Geometry: final body of the model. Coordinates: model frame, mm. A direction names the side the tool comes from. Give positions to 0.01 mm unless a question says otherwise; leave off trailing zeros. Write each loop counter-clockwise with the first axis right and the second up, starting at its lowest first coordinate (ties: lowest second). Pieces come first, ordered by that corner, then holes. Notation, with made-up numbers: (47, 41.5) -> (85, 41.5) arc R26 ccw to (85, 71.5) -> close; hole circle Ø8 at (-17.5, 33). An arc over 180 degrees is marked (long way). Answer in a Markdown table with one row per item. Add a question column.
from build123d import *

# Parameters (mm, degrees)
SKETCH_1_R               = 1.5
EXTRUDE_1_DEPTH          = 2
SKETCH_3_W               = 250
SKETCH_3_H               = 20
CUT_EXTRUDE_2_DEPTH      = 138.815093513
CUT_EXTRUDE_3_DEPTH      = 138.815093513
CUT_EXTRUDE_3_DEPTH_BACK = 138.815093513
CUT_EXTRUDE_4_DEPTH      = 138.815093513


with BuildPart() as part:
    # 草图1 → 凸台-拉伸1 (new body)
    with BuildSketch(Plane.XY):
        Polygon((-77, 30), (-77, 0), (77, 0), (77, 30), (125, 30), (125, 0), (67, -58), (-67, -58), (-125, 0), (-125, 30), align=None)
        with Locations((-121, 25)):
            Circle(SKETCH_1_R, mode=Mode.SUBTRACT)
        with Locations((-81, 25)):
            Circle(SKETCH_1_R, mode=Mode.SUBTRACT)
        with Locations((-81, 5)):
            Circle(SKETCH_1_R, mode=Mode.SUBTRACT)
        with Locations((-121, 5)):
            Circle(SKETCH_1_R, mode=Mode.SUBTRACT)
        with Locations(Location((121, 5, 0), (0, 0, 180))):
            Circle(SKETCH_1_R, mode=Mode.SUBTRACT)
        with Locations(Location((81, 5, 0), (0, 0, 180))):
            Circle(SKETCH_1_R, mode=Mode.SUBTRACT)
        with Locations(Location((81, 25, 0), (0, 0, 180))):
            Circle(SKETCH_1_R, mode=Mode.SUBTRACT)
        with Locations(Location((121, 25, 0), (0, 0, 180))):
            Circle(SKETCH_1_R, mode=Mode.SUBTRACT)
    extrude(amount=EXTRUDE_1_DEPTH)

    # 草图3 → 切除-拉伸2 (cut, through all)
    with BuildSketch(Plane.XY.offset(2)):
        with Locations((0, 20)):
            Rectangle(SKETCH_3_W, SKETCH_3_H)
    extrude(amount=-CUT_EXTRUDE_2_DEPTH, mode=Mode.SUBTRACT)

    # 草图4 → 切除-拉伸3 (cut, two sides: drawn at the far end of the back side and taken through both)
    with BuildSketch(Plane.XY.offset(2).offset(-CUT_EXTRUDE_3_DEPTH_BACK)):
        with BuildLine():
            Line((-91.226136393, -12.560660172), (-69.560660172, -34.226136393))
            ThreePointArc((-69.560660172, -34.226136393), (-67.925974851, -34.55129552), (-67, -33.165476221))
            Line((-67, -33.165476221), (-67, -11.5))
            ThreePointArc((-67, -11.5), (-67.439339828, -10.439339828), (-68.5, -10))
            Line((-68.5, -10), (-90.165476221, -10))
            ThreePointArc((-90.165476221, -10), (-91.55129552, -10.925974851), (-91.226136393, -12.560660172))
        make_face()
        with BuildLine():
            Line((68.5, -10), (90.165476221, -10))
            ThreePointArc((90.165476221, -10), (91.55129552, -10.925974851), (91.226136393, -12.560660172))
            Line((91.226136393, -12.560660172), (69.560660172, -34.226136393))
            ThreePointArc((69.560660172, -34.226136393), (67.925974851, -34.55129552), (67, -33.165476221))
            Line((67, -33.165476221), (67, -11.5))
            ThreePointArc((67, -11.5), (67.439339828, -10.439339828), (68.5, -10))
        make_face()
        with BuildLine():
            Line((-5.5, -36.928047473), (-5.5, -44.428047473))
            ThreePointArc((-5.5, -44.428047473), (-8, -46.928047473), (-10.5, -44.428047473))
            Line((-10.5, -44.428047473), (-10.5, -24.428047473))
            ThreePointArc((-10.5, -24.428047473), (-8, -21.928047473), (-5.5, -24.428047473))
            Line((-5.5, -24.428047473), (-5.5, -31.928047473))
            Line((-5.5, -31.928047473), (5.5, -31.928047473))
            Line((5.5, -31.928047473), (5.5, -24.428047473))
            ThreePointArc((5.5, -24.428047473), (8, -21.928047473), (10.5, -24.428047473))
            Line((10.5, -24.428047473), (10.5, -44.428047473))
            ThreePointArc((10.5, -44.428047473), (8, -46.928047473), (5.5, -44.428047473))
            Line((5.5, -44.428047473), (5.5, -36.928047473))
            Line((5.5, -36.928047473), (-5.5, -36.928047473))
        make_face()
    extrude(amount=CUT_EXTRUDE_3_DEPTH + CUT_EXTRUDE_3_DEPTH_BACK, mode=Mode.SUBTRACT)

    # 草图5 → 切除-拉伸4 (cut, through all)
    with BuildSketch(Plane.XY.offset(2)):
        with BuildLine():
            Line((-121, 6.75), (-81, 6.75))
            ThreePointArc((-81, 6.75), (-79.25, 5), (-81, 3.25))
            Line((-81, 3.25), (-121, 3.25))
            ThreePointArc((-121, 3.25), (-122.75, 5), (-121, 6.75))
        make_face()
        with BuildLine():
            Line((81, 6.75), (121, 6.75))
            ThreePointArc((121, 6.75), (122.75, 5), (121, 3.25))
            Line((121, 3.25), (81, 3.25))
            ThreePointArc((81, 3.25), (79.25, 5), (81, 6.75))
        make_face()
    extrude(amount=-CUT_EXTRUDE_4_DEPTH, mode=Mode.SUBTRACT)


solid = part.part
Q1. Pull-direction query (X, two-part tool) for faces 1 (the flat face through (-96, -29, 1)), 2 (the flat face through (-80.545, -23.242, 0.986)), 3 (the flat face through (2, -24, 2)); classes: +X half, -X half, draft (parallel to the pull), parting line (faces both ways), or undercut.
Q2. Access query for faces 4 (the flat face through (80.545, -23.242, 0.986)), 5 (the flat face through (2, -24, 0)). Directions: +Z, -Z, +X, -X, +Y, -Y. A direction counts if a zero-diameter tool reaches every point of the face in a straight line with its end or side. Return the directions, or none.
Q3. Contact query for flat-ended pins moving along their axis: pin 1 Ø1 at (x, z) = (76, 1.5) entering from -Y; pin 2 Ø0.6 at (y, z) = (-29, 1.5) entering from -X; pin 3 Ø1 at (x, z) = (25.5, 1.5) entering from +Y; pin 4 Ø5 at (x, y) = (7.5, -30) entering from +Z. Output: stop coordinate, or through.
Q4. Section B-B on z = 1.55. Count the separate pieces of the cut face and the enclosed holes in it, and give its area (3 significant figures).
Q5. Section A-A on x = -8. Return loops of the section in (y, z), and give its area (3 significant figures).
Q6. Line query: probe 1 along X at (y, z) = (-23.5, 0.8); probe 2 along X at (y, z) = (-13, 1.75); probe 3 along X at (y, z) = (-15, 0.55). Output: solid intervals per line, ascending. Write a range as from..to.
Checks:
| question | item | result |
|---|---|---|
| 1 | face 1 | -X half |
| 1 | face 2 | undercut |
| 1 | face 3 | draft |
| 2 | face 4 | +Z, -Z |
| 2 | face 5 | -Z, +X, -X, +Y, -Y |
| 3 | pin 1 | y = -49.5 |
| 3 | pin 2 | x = -96.3 |
| 3 | pin 3 | y = 0 |
| 3 | pin 4 | z = 2 |
| 4 | separate pieces | 1 |
| 4 | enclosed holes | 5 |
| 4 | area | 10,800 mm^2 |
| 5 | outline | (-58, 0) -> (-46.93, 0) -> (-46.93, 2) -> (-58, 2) -> close; (-21.93, 0) -> (0, 0) -> (0, 2) -> (-21.93, 2) -> close |
| 5 | area | 66.0 mm^2 |
| 6 | probe 1 | -101.5..-80.29, -67..-10.32, -5.68..5.68, 10.32..67, 80.29..101.5 |
| 6 | probe 2 | -112..-90.79, -67..67, 90.79..112 |
| 6 | probe 3 | -110..-88.79, -67..67, 88.79..110 |
